Design review of the part built by this model. Coordinates are the model's own, in mm. Face numbers are marked on the shaded views. Coordinates: 2 decimals unless noted, no trailing zeros. One line per item, written item: value.
Autodesk Inventor part; units mm, degrees
ref_plane "YZ Plane" through (0, 0, 0) normal (1, 0, 0) x (0, 1, 0)
ref_plane "XZ Plane" through (0, 0, 0) normal (0, 1, 0) x (-1, 0, 0)
ref_plane "XY Plane" through (0, 0, 0) normal (0, 0, 1) x (1, 0, 0)
sketch "Sketch1" plane through (0, 0, 0) normal (0, 1, 0) x (-1, 0, 0)
  circle A0 centre (0, 0) radius 32.5
  circle A1 centre (0, 0) radius 35.5
  dimension "d0" = 65
  dimension "d1" = 71
extrude "Extrusion1" add sketch "Sketch1" along normal blind 8
extrude "Extrusion2" add sketch "Sketch1" along normal blind 3 contours A0
fillet "Fillet1" radius 2 2 edges at (35.5, 0, 0) (32.5, 3, 0)
fillet "Fillet2" radius 1.5 2 edges at (32.5, 8, 0) (35.5, 8, 0)
sketch "Sketch2" plane through (0, 3, 0) normal (0, 1, 0) x (1, 0, 0)
  circle A0 centre (0, 0) radius 0.25
  circle A1 centre (0, 0) radius 2.5
  circle A2 centre (0, 2) radius 0.5
  line L0 (-0.5, 2) -> (-0.5, 1.5) construction
  line L1 (-0.5, 1.5) -> (-0.25, 0.892563) construction
  line L2 (-0.25, 0.892563) -> (0, 0.421283) construction
  spline S0 degree 3 poles (-0.5, 2) (-0.5, 1.5) (-0.25, 0.892563) (0, 0.421283) knots 1 1 1 1 2 2 2 2
  line L3 (-0.5, 1.5) -> (0.5, 1.5)
  line L4 (-0.25, 0.892563) -> (0.25, 0.892563)
  line L5 (0.5, 2) -> (0.5, 1.5) construction
  line L6 (0.5, 1.5) -> (0.25, 0.892563) construction
  line L7 (0.25, 0.892563) -> (0, 0.421283) construction
  spline S1 degree 3 poles (0.5, 2) (0.5, 1.5) (0.25, 0.892563) (0, 0.421283) knots 1 1 1 1 2 2 2 2
  dimension "d12" = 0.5
  dimension "d13" = 5
sketch "Sketch2 outline for Extrusion4" plane through (0, 3, 0) normal (0, 1, 0) x (1, 0, 0)
  circle A0 centre (0, 0) radius 0.25
  spline S0 degree 3 poles (0.5, 2) (0.5, 1.5) (0.25, 0.892563) (0, 0.421283) knots 0 0 0 0 1 1 1 1
  spline S1 degree 3 poles (-0.5, 2) (-0.5, 1.5) (-0.25, 0.892563) (0, 0.421283) knots 0 0 0 0 1 1 1 1
  arc A1 (0.5, 2) -> (-0.5, 2) centre (0, 2) ccw
extrude "Extrusion4" add sketch "Sketch2 outline for Extrusion4" along normal blind 0.5
pattern_circular "Circular Pattern1" count 9 over 360 about axis through (0, -10, 0) along (0, 1, 0) of "Extrusion4"
properties part number "Orchid Coaster V5"
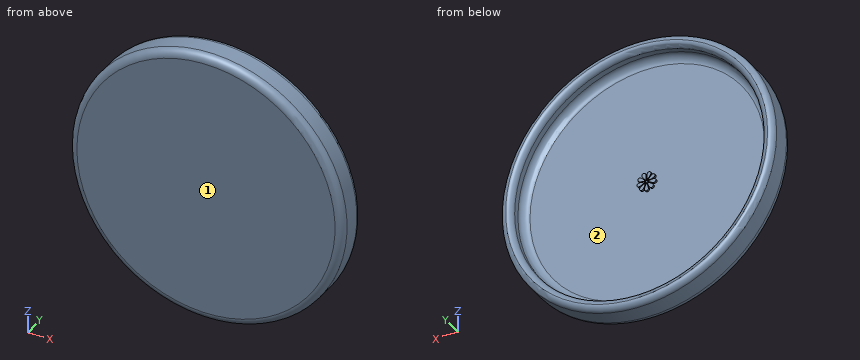
1. Wall thickness on line 1 along Z through (x, y) = (0, 5.8); line 2 along Y through (x, z) = (-11.5, 17); line 3 along Z through (x, y) = (3, 5.5): over which ranges is each line inside the solid? List them lowest first.
Answer block:
line 1: z = -35.5 to -32.5, 32.5 to 35.5
line 2: y = 0 to 3
line 3: z = -35.37 to -32.36, 32.36 to 35.37
2. Mouldability with a two-part tool opening along Z and no side actions: class the marked faces 1 and 2 as released by +Z, released by -Z, zero draft, split by the parting line, or undercut.
Answer block:
face 1: zero draft
face 2: undercut
3. Insertion check: pin 1 Ø2 at (x, z) = (17, 17.5) entering from +Y; pin 2 Ø1 at (x, z) = (-1, 1) entering from +Y; pin 3 Ø4 at (x, y) = (-24.5, 5.5) entering from -Z. Each pin has a flat end and moves straight along its axis. Give the tip position at first contact, or say it passes through.
Answer block:
pin 1: stops at y = 3
pin 2: stops at y = 3.5
pin 3: stops at z = -27.46
